```python
from build123d import *

# Parameters (mm, degrees)
ESQUISSE5_R        = 3.4
ESQUISSE5_R_2      = 2.6
BOSS_EXTRU_1_DEPTH = 27
ESQUISSE6_R        = 3.4
BOSS_EXTRU_2_DEPTH = 0.5
BOSS_EXTRU_4_START = 1.5
BOSS_EXTRU_4_DEPTH = 1.9
BOSS_EXTRU_5_DEPTH = 4


with BuildPart() as part:
    # Esquisse5 → Boss.-Extru.1 (new body)
    with BuildSketch(Plane.XY):
        Circle(ESQUISSE5_R)
        Circle(ESQUISSE5_R_2, mode=Mode.SUBTRACT)
    extrude(amount=BOSS_EXTRU_1_DEPTH)

    # Esquisse6 → Boss.-Extru.2 (add)
    with BuildSketch(Plane.XY.offset(27)):
        Circle(ESQUISSE6_R)
    extrude(amount=BOSS_EXTRU_2_DEPTH)



with BuildPart() as body_2:
    # Esquisse9 → Boss.-Extru.4 (new body)
    with BuildSketch(Plane(origin=(0, 0, 0), x_dir=(0, 0, -1), z_dir=(1, 0, 0)).offset(BOSS_EXTRU_4_START)):
        with BuildLine():
            Line((-4, -3.4), (-4, -13.5))
            ThreePointArc((-4, -13.5), (-2, -15.5), (0, -13.5))
            Line((0, -13.5), (0, -3.4))
            Line((0, -3.4), (-4, -3.4))
        make_face()
        with BuildLine():
            ThreePointArc((-1.35, -8.5), (-2, -7.85), (-2.65, -8.5))
            Line((-2.65, -8.5), (-2.65, -13.5))
            ThreePointArc((-2.65, -13.5), (-2, -14.15), (-1.35, -13.5))
            Line((-1.35, -13.5), (-1.35, -8.5))
        make_face(mode=Mode.SUBTRACT)
    extrude(amount=BOSS_EXTRU_4_DEPTH)


with BuildPart() as part_1:
    add(part.part)

    add(body_2.part)  # Boss.-Extru.5 merges body 2
    # Esquisse10 → Boss.-Extru.5 (add)
    with BuildSketch(Plane(origin=(0, 0, 0), x_dir=(-1, 0, 0), z_dir=(0, 0, -1))):
        with BuildLine():
            Line((-3.4, -3.4), (0, -3.4))
            ThreePointArc((0, -3.4), (-2.404163056, -2.404163056), (-3.4, 0))
            Line((-3.4, 0), (-3.4, -3.4))
        make_face()
    extrude(amount=-BOSS_EXTRU_5_DEPTH)


solid = part_1.part
```
Can you work these out from the model? Positions are in its coordinate system, mm. A direction names the side the tool comes from. Coordinates: 2 decimals unless noted, no trailing zeros. Order: outer loops, then holes, each group sorted by start corner. A loop starts at its lowest first (then second) coordinate and runs counter-clockwise, first axis right, second up. Notation, with made-up numbers: (-0.5, 38) - (39.5, 38) arc R14 ccw to (39.5, 47) - close; hole circle Ø8 at (-31.75, 68). An arc over 180 degrees is marked (long way). Answer in a Markdown table with one row per item.
1. For faces 1 (the flat face through (0, 0, 27)), 2 (the flat face through (1.5, -9, 3)), 3 (the cylindrical face through (-2.506, 2.298, 13.558)), which set-ups out of +Z, -Z, +X, -X, +Y, -Y let a thin tool reach every point of the face, with its end or its side?
Reply:
| item | result |
|---|---|
| face 1 | -Z |
| face 2 | +Z, -Z, -X, -Y |
| face 3 | +Z |
2. Suppose I cut it at D-D (x = -2.25). Please give me the cut outline in (y, z).
Reply:
| item | result |
|---|---|
| outline | (-2.55, 0) - (-1.3, 0) - (-1.3, 27) - (1.3, 27) - (1.3, 0) - (2.55, 0) - (2.55, 27.5) - (-2.55, 27.5) - close |
3. Suppose I cut it at C-C (x = 3). Please give me the cut outline in (y, z).
Reply:
| item | result |
|---|---|
| outline | (-13.5, 0) - (1.6, 0) - (1.6, 27.5) - (-1.6, 27.5) - (-1.6, 4) - (-13.5, 4) arc R2 ccw to start; hole (-13.5, 1.35) - (-8.5, 1.35) arc R0.65 ccw to (-8.5, 2.65) - (-13.5, 2.65) arc R0.65 ccw to start |
4. For pin 1 (1.5 mm diameter, centred on x = -2, z = 4.5, fed in from -Y); pin 2 (1.5 mm diameter, centred on x = 2.5, y = -12, fed in from +Z); pin 3 (1.2 mm diameter, centred on y = -11, z = 1.5, fed in from -X), each with a flat end and sliding along its axis, tell me the tip position at first contact or that it passes through.
Reply:
| item | result |
|---|---|
| pin 1 | stops at y = -3.16 |
| pin 2 | stops at z = 4 |
| pin 3 | stops at x = 1.5 |
5. Suppose I cut it at B-B (y = -12.25). Please give me the cut outline in (x, z), and give its area (3 significant figures).
Reply:
| item | result |
|---|---|
| outline | (1.5, 0) - (3.4, 0) - (3.4, 1.35) - (1.5, 1.35) - close; (1.5, 2.65) - (3.4, 2.65) - (3.4, 4) - (1.5, 4) - close |
| area | 5.13 mm^2 |
6. If we mould it in two halves opening along Z, with no side actions, what happens to faces 4 (the flat face through (2, -8, 4)), 5 (the cylindrical face through (-0.338, 2.578, 13.311)), 6 (the flat face through (2, -11, 2.65))? For each: pulls with the +Z half, pulls with the -Z half, needs draft (parallel to the pull), parting line crosses it, or undercut.
Reply:
| item | result |
|---|---|
| face 4 | pulls with the +Z half |
| face 5 | needs draft |
| face 6 | undercut |
7. Suppose I cut it at A-A (z = 2). Please give me the cut outline in (x, y).
Reply:
| item | result |
|---|---|
| outline | (0, -3.4) - (1.5, -3.4) - (1.5, -7.85) - (3.4, -7.85) - (3.4, 0) arc R3.4 ccw (long way) to start; (1.5, -15.5) - (3.4, -15.5) - (3.4, -14.15) - (1.5, -14.15) - close; hole circle Ø5.2 at (0, 0) |
8. If I drill on line 1 along Z through (x, y) = (2.5, -9.5); line 2 along Y through (x, z) = (0, 10.25); line 3 along Z through (x, y) = (1.75, -0.25), over which ranges is the centre line in solid material (lowest first)?
Reply:
| item | result |
|---|---|
| line 1 | z = 0 to 1.35, 2.65 to 4 |
| line 2 | y = -3.4 to -2.6, 2.6 to 3.4 |
| line 3 | z = 27 to 27.5 |
